Design review of the part shown in the three views and the two pictorial views. Dimensions are in mm from the part's minimum x, y and z. A direction names the side the tool comes from. Round coordinates to 2 decimals unless told otherwise and drop trailing zeros. Write each loop counter-clockwise with the first axis right and the second up, starting at its lowest first coordinate (ties: lowest second). Pieces come first, ordered by that corner, then holes. Notation, with made-up numbers: (-22.5, -38) -> (15.5, -38) arc R34 cw to (15.5, -4) -> close; hole circle Ø8 at (-20.5, -35). An arc over 180 degrees is marked (long way). Return JSON: item names as keys, results as strings. Group by question number.
1. Tool access review of the marked faces 1, 2 and 3: name each direction out of +Z, -Z, +X, -X, +Y, -Y from which nothing blocks a thin tool from reaching the whole face with its end or side.
2. Clearance check with flat-ended pins moving along their axes: P1, Ø1.5, axis at x = 8.5, z = 3, coming from the +Y side; P2, Ø5, axis at x = 7, y = 27.5, coming from the +Z side. State where each tip first meets the part, or that it passes through.
3. Mouldability with a two-part tool opening along Y and no side actions: class the marked faces 4, 5 and 6 as pulls with the +Y half, pulls with the -Y half, needs draft (parallel to the pull), parting line crosses it, or undercut.
4. Take a section at C-C, the plane z = 2.6. Write out the cut boundary in (x, y) (3 decimals), then the cut area to 3 significant figures.
5. Take a section at D-D, the plane y = 12.75. Write out the cut boundary in (x, z) (3 decimals).
6. Take a section at B-B, the plane x = 6.5. Write out the cut boundary in (y, z).
7. Take a section at A-A, the plane y = 26.4. Write out the cut boundary in (x, z) (3 decimals).
8. For line 1 along Y through (x, z) = (6, 1.9); line 2 along Z through (x, y) = (2.25, 27.5); line 3 along Y through (x, z) = (5, 2.2), list the stretches that pass through material, from the lowest coordinate up. Write a range as from..to.
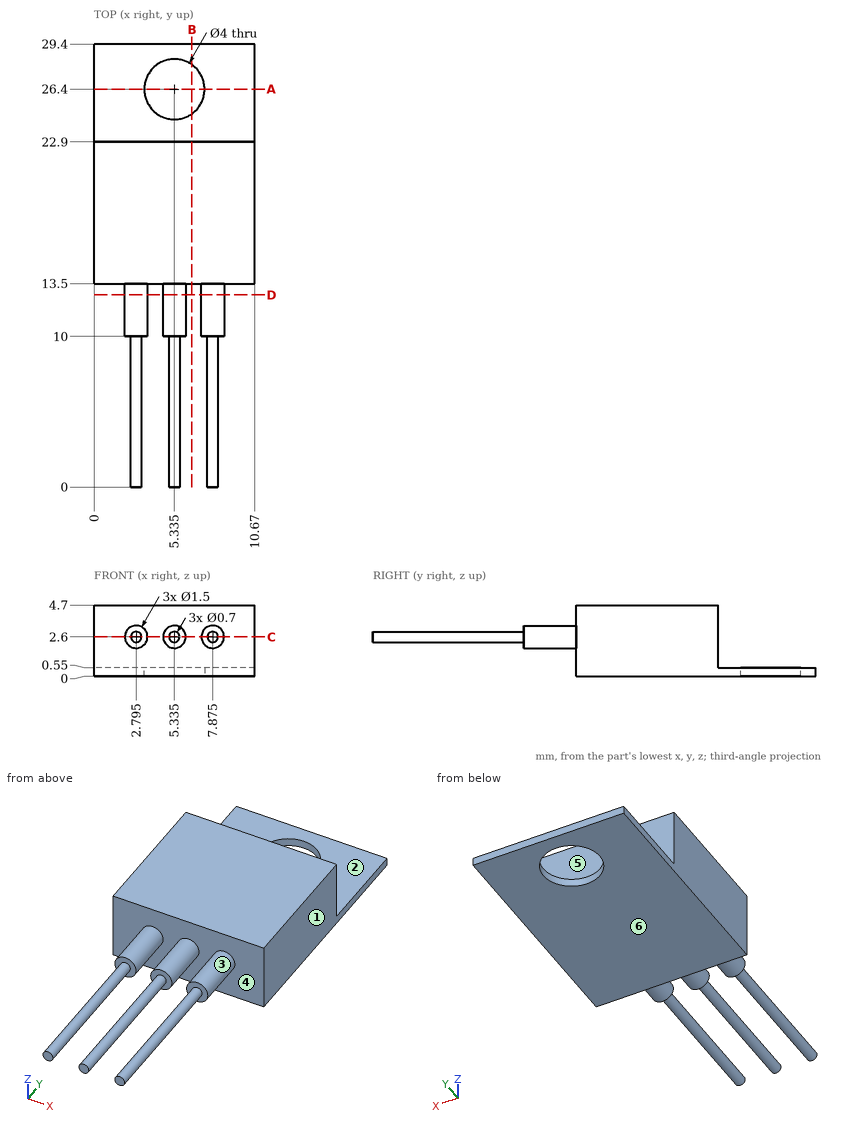
Output:
{
 "1": {"face 1": "+Z, -Z, +X, +Y, -Y", "face 2": "+Z, +X, -X, +Y", "face 3": "-Y"},
 "2": {"P1": "stops at y = 22.9", "P2": "stops at z = 0.55"},
 "3": {"face 4": "pulls with the -Y half", "face 5": "pulls with the +Y half", "face 6": "needs draft"},
 "4": {"outline": "(0, 13.5) -> (2.045, 13.5) -> (2.045, 10) -> (2.445, 10) -> (2.445, 0) -> (3.145, 0) -> (3.145, 10) -> (3.545, 10) -> (3.545, 13.5) -> (4.585, 13.5) -> (4.585, 10) -> (4.985, 10) -> (4.985, 0) -> (5.685, 0) -> (5.685, 10) -> (6.085, 10) -> (6.085, 13.5) -> (7.125, 13.5) -> (7.125, 10) -> (7.525, 10) -> (7.525, 0) -> (8.225, 0) -> (8.225, 10) -> (8.625, 10) -> (8.625, 13.5) -> (10.67, 13.5) -> (10.67, 22.9) -> (0, 22.9) -> close", "area": "137 mm^2"},
 "5": {"outline": "circle Ø1.5 at (2.795, 2.6); circle Ø1.5 at (5.335, 2.6); circle Ø1.5 at (7.875, 2.6)"},
 "6": {"outline": "(13.5, 0) -> (24.77, 0) -> (24.77, 0.55) -> (22.9, 0.55) -> (22.9, 4.7) -> (13.5, 4.7) -> close; (28.03, 0) -> (29.4, 0) -> (29.4, 0.55) -> (28.03, 0.55) -> close"},
 "7": {"outline": "(0, 0) -> (3.335, 0) -> (3.335, 0.55) -> (0, 0.55) -> close; (7.335, 0) -> (10.67, 0) -> (10.67, 0.55) -> (7.335, 0.55) -> close"},
 "8": {"line 1": "y = 13.5..22.9", "line 2": "z = 0..0.55", "line 3": "y = 10..22.9"}
}
